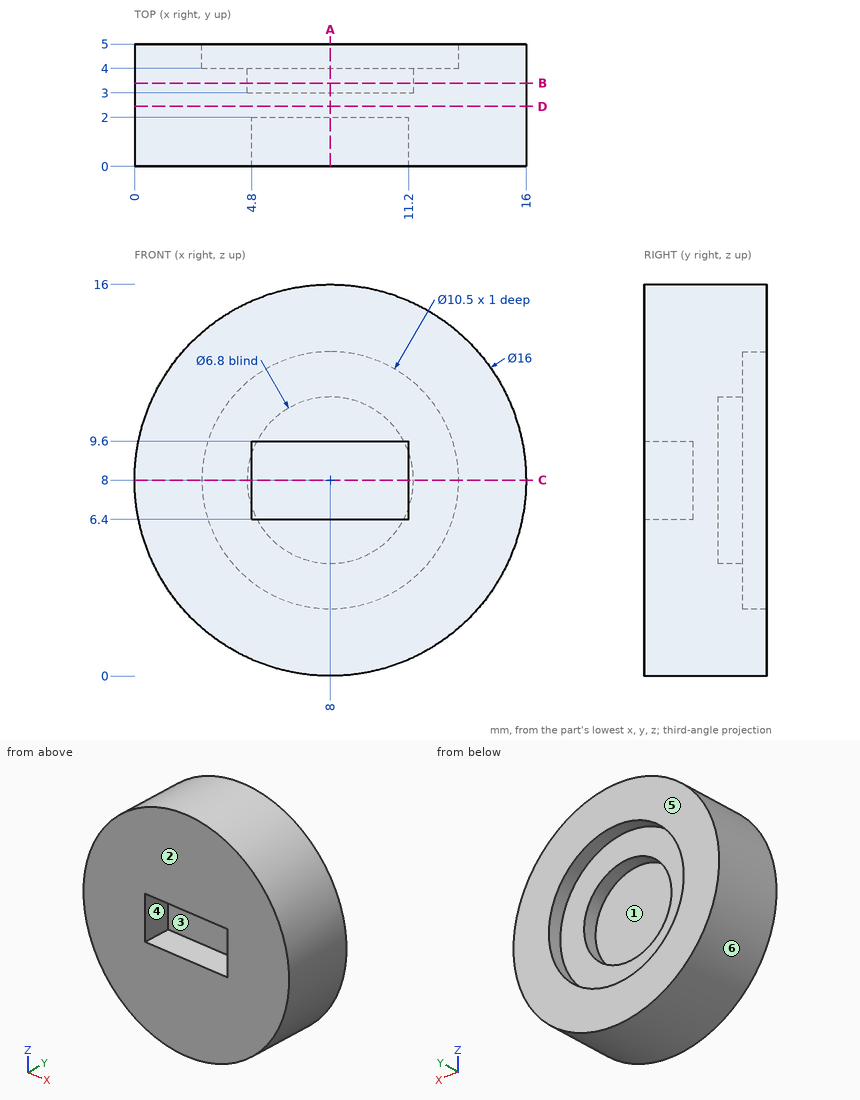
Answer from the drawing. Dimensions are ordinates in mm from the lowest x, y and z of the part. A direction names the side the tool comes from. Coordinates: 2 decimals unless noted, no trailing zeros. Loops run counter-clockwise (first coordinate to the right, second up) from the corner with the lowest first, then second, coordinate; pieces in that order, holes last. Notation, with made-up numbers: (-24.5, 26) -> (3.5, 26) arc R15 cw to (3.5, 44) -> close; hole circle Ø5 at (-4.5, -40). An arc over 180 degrees is marked (long way). Answer in a Markdown table with one row per item.
Item 1: A cutting plane is placed at B-B on y = 3.4. Determine the outline of the cut face in (x, z), plus the area to 3 significant figures.
Returned:
| item | result |
|---|---|
| outline | circle Ø16 at (8, 8); hole circle Ø6.8 at (8, 8) |
| area | 165 mm^2 |
Item 2: For a pull along Z with two mould halves and no side action, classify the marked faces 4, 5 and 6 as released by +Z, released by -Z, zero draft, split by the parting line, or undercut.
Returned:
| item | result |
|---|---|
| face 4 | undercut |
| face 5 | zero draft |
| face 6 | split by the parting line |
Item 3: Straight lines are drawn through the part: line 1 along X through (y, z) = (4.65, 8); line 2 along X through (y, z) = (3.6, 8); line 3 along Y through (x, z) = (7.25, 10). For each, find the intervals that lie inside material, in ascending order. Write a range as [from, to].
Returned:
| item | result |
|---|---|
| line 1 | x = [0, 2.75], [13.25, 16] |
| line 2 | x = [0, 4.6], [11.4, 16] |
| line 3 | y = [0, 3] |
Item 4: A cutting plane is placed at C-C on z = 8. Determine the outline of the cut face in (x, y), plus the area to 3 significant figures.
Returned:
| item | result |
|---|---|
| outline | (0, 0) -> (4.8, 0) -> (4.8, 2) -> (11.2, 2) -> (11.2, 0) -> (16, 0) -> (16, 5) -> (13.25, 5) -> (13.25, 4) -> (11.4, 4) -> (11.4, 3) -> (4.6, 3) -> (4.6, 4) -> (2.75, 4) -> (2.75, 5) -> (0, 5) -> close |
| area | 49.9 mm^2 |
Item 5: A cutting plane is placed at D-D on y = 2.45. Determine the outline of the cut face in (x, z), plus the area to 3 significant figures.
Returned:
| item | result |
|---|---|
| outline | circle Ø16 at (8, 8) |
| area | 201 mm^2 |
Item 6: For the marked faces 1, 2 and 3, determine the directions among +Z, -Z, +X, -X, +Y, -Y from which every point of the face is accessible in a straight line to the end or side of a thin tool.
Returned:
| item | result |
|---|---|
| face 1 | +Y |
| face 2 | +Z, -Z, +X, -X, -Y |
| face 3 | -Y |
Item 7: Each of these flat-tipped pins is pushed along its axis until it touches: P1, Ø1.6, axis at x = 6.5, y = 1.5, coming from the -Z side; P2, Ø0.6, axis at y = 1, z = 7, coming from the +X side; P3, Ø1, axis at x = 4.5, y = 3, coming from the -Z side. Where does it stop, or does it pass through?
Returned:
| item | result |
|---|---|
| P1 | stops at z = 0.03 |
| P2 | stops at x = 15.97 |
| P3 | stops at z = 0.58 |
Item 8: A cutting plane is placed at A-A on x = 8. Determine the outline of the cut face in (y, z).
Returned:
| item | result |
|---|---|
| outline | (0, 0) -> (5, 0) -> (5, 2.75) -> (4, 2.75) -> (4, 4.6) -> (3, 4.6) -> (3, 11.4) -> (4, 11.4) -> (4, 13.25) -> (5, 13.25) -> (5, 16) -> (0, 16) -> (0, 9.6) -> (2, 9.6) -> (2, 6.4) -> (0, 6.4) -> close |
